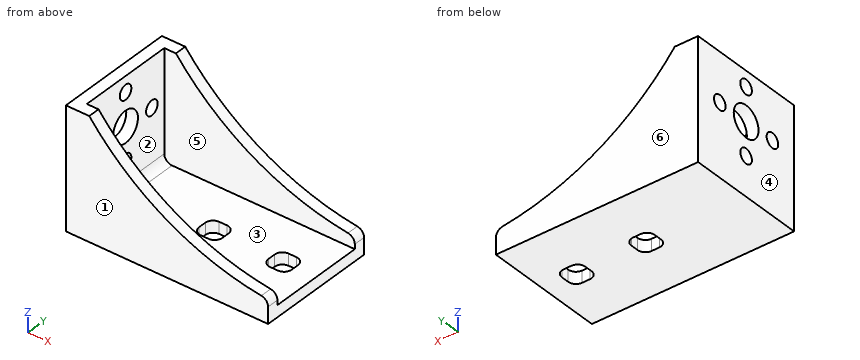
Autodesk Inventor part; units mm, degrees
ref_plane "YZ Plane" through (0, 0, 0) normal (1, 0, 0) x (0, 1, 0)
ref_plane "XZ Plane" through (0, 0, 0) normal (0, 1, 0) x (-1, 0, 0)
ref_plane "XY Plane" through (0, 0, 0) normal (0, 0, 1) x (1, 0, 0)
sketch "Sketch1" plane through (0, 0, 0) normal (0, 0, 1) x (1, 0, 0)
  line L0 (0, 0) -> (52, 0)
  line L1 (52, 0) -> (52, 31)
  line L2 (52, 31) -> (0, 31)
  line L3 (0, 31) -> (0, 0)
  line L4 (24.7, 18.5) -> (26.7, 18.5)
  line L5 (28.7, 16.5) -> (28.7, 14.5)
  line L6 (26.7, 12.5) -> (24.7, 12.5)
  line L7 (22.7, 14.5) -> (22.7, 16.5)
  arc A0 (22.7, 14.5) -> (24.7, 12.5) centre (24.7, 14.5) ccw
  arc A1 (24.7, 18.5) -> (22.7, 16.5) centre (24.7, 16.5) ccw
  arc A2 (28.7, 16.5) -> (26.7, 18.5) centre (26.7, 16.5) ccw
  arc A3 (26.7, 12.5) -> (28.7, 14.5) centre (26.7, 14.5) ccw
  line L8 (42.542, 18.5) -> (44.542, 18.5)
  line L9 (46.542, 16.5) -> (46.542, 14.5)
  line L10 (44.542, 12.5) -> (42.542, 12.5)
  line L11 (40.542, 14.5) -> (40.542, 16.5)
  arc A4 (40.542, 14.5) -> (42.542, 12.5) centre (42.542, 14.5) ccw
  arc A5 (42.542, 18.5) -> (40.542, 16.5) centre (42.542, 16.5) ccw
  arc A6 (46.542, 16.5) -> (44.542, 18.5) centre (44.542, 16.5) ccw
  arc A7 (44.542, 12.5) -> (46.542, 14.5) centre (44.542, 14.5) ccw
  point P0 (28.7, 12.5)
  point P1 (28.7, 18.5)
  point P2 (22.7, 12.5)
  point P3 (22.7, 15.5)
  point P4 (0, 15.5)
  point P5 (46.542, 12.5)
  point P6 (46.542, 18.5)
  point P7 (40.542, 12.5)
  point P8 (40.542, 15.5)
  point P9 (28.7, 15.5)
  dimension "d0" = 52
  dimension "d1" = 31
  dimension "d2" = 6
  dimension "d3" = 6
  dimension "d4" = 2
  dimension "d5" = 22.7
  dimension "d6" = 6
  dimension "d7" = 6
  dimension "d8" = 2
  dimension "d9" = 5.458
extrude "Extrusion1" add sketch "Sketch1" along normal blind 3
sketch "Sketch2" plane through (0, 0, 3) normal (0, 0, 1) x (1, 0, 0)
  line L0 (0, 31) -> (0, 0) construction
  line L1 (52, 31) -> (0, 31) construction
  line L2 (0, 0) -> (3, 0)
  line L3 (3, 0) -> (3, 31)
  line L4 (3, 31) -> (0, 31)
  line L5 (0, 31) -> (0, 0)
  dimension "d12" = 3
extrude "Extrusion2" add sketch "Sketch2" along normal blind 28
fillet "Fillet1" radius 2 1 edges at (3, 15.5, 3)
sketch "Sketch4" plane through (0, 0, 0) normal (-1, 0, 0) x (0, 0, 1)
  point P0 (0, 0)
  point P1 (18.5, 15.5)
  point P2 (31, 15.5)
  dimension "d40" = 12.5
hole "Hole1" at (0, 15.5, 18.5) direction (1, 0, 0) diameter 8 end through all
sketch "Sketch5" plane through (0, 0, 0) normal (-1, 0, 0) x (0, 0, 1)
  line L0 (0, 31) -> (0, 0) construction
  circle A0 centre (18.5, 15.5) radius 4 construction
  point P0 (18.5, 7)
  dimension "d28" = 8.5
hole "Hole2" at (0, 7, 18.5) direction (1, 0, 0) diameter 3.74 end through all
pattern_circular "Circular Pattern1" count 4 over 360 about axis through (68.0147, 15.5, 18.5) along (-1, 0, 0) of "Hole2"
sketch "Sketch7" plane through (3, 0, 31) normal (1, 0, 0) x (0, 0, -1)
  line L0 (0, 0) -> (31, 0)
  line L1 (31, 0) -> (31, 3)
  line L2 (31, 3) -> (0, 3)
  line L3 (0, 3) -> (0, 0)
  line L4 (0, 28) -> (31, 28)
  line L5 (31, 28) -> (31, 31)
  line L6 (31, 31) -> (0, 31)
  line L7 (0, 31) -> (0, 28)
  point P0 (31, 0)
  dimension "d41" = 3
  dimension "d42" = 3
extrude "Extrusion4" add sketch "Sketch7" along normal up to surface (49 mm away)
sketch "Sketch8" plane through (0, 0, 0) normal (0, -1, 0) x (1, 0, 0)
  line L0 (3, 31) -> (6, 31) construction
  line L1 (52, 3) -> (52, 6) construction
  arc A0 (6, 31) -> (52, 6) centre (58.6945, 73.1378) ccw
  line L2 (6, 31) -> (52, 31)
  line L3 (52, 31) -> (52, 6)
  point P0 (0, 0)
  dimension "d45" = 3
  dimension "d46" = 3
  dimension "d47" = 67.4708
extrude "Extrusion5" cut sketch "Sketch8" against normal up to surface (31 mm away)
fillet "Fillet2" radius 2 2 edges at (52, 1.5, 6) (52, 29.5, 6)
properties part number "sujetador del motor"
Check sheet for the modelled part. Datum: model origin and axes. Units: mm. Face numbers are marked on the shaded views. A direction names the side the tool comes from. Give positions to 0.01 mm unless a question says otherwise; leave off trailing zeros. Write each loop counter-clockwise with the first axis right and the second up, starting at its lowest first coordinate (ties: lowest second). Pieces come first, ordered by that corner, then holes. Notation, with made-up numbers: (-31.5, 37) -> (2.5, 37) arc R16 cw to (2.5, 53) -> close; hole circle Ø8 at (-16, -18.5). An arc over 180 degrees is marked (long way). Write item = value, one per line.
Item 1: Gauge pin test, flat ends, axial feed: pin 1 (5 mm diameter, centred on y = 7, z = 18.5, fed in from -X); pin 2 (1 mm diameter, centred on x = 42.5, y = 5.5, fed in from +Z); pin 3 (7.5 mm diameter, centred on y = 16.5, z = 16, fed in from +X); pin 4 (3 mm diameter, centred on y = 15.5, z = 27, fed in from -X). Record the tip position at first contact, or that the pin passes through.
Output:
pin_1 = 0
pin_2 = 3
pin_3 = 3
pin_4 = through
Item 2: Tool access check on the marked faces 1 and 2. Record the directions out of +Z, -Z, +X, -X, +Y, -Y that give a thin tool (end or side, any length) a straight path to the whole face; none if there is none.
Output:
face_1 = +Z, -Z, +X, -X, -Y
face_2 = +Z, +X
Item 3: Sectioned sample at B-B on y = 15.5. Record the boundary of the cut face in (x, z), and give its area (3 significant figures).
Output:
outline = (0, 0) -> (22.7, 0) -> (22.7, 3) -> (5, 3) arc R2 cw to (3, 5) -> (3, 8.13) -> (0, 8.13) -> close; (0, 11.87) -> (3, 11.87) -> (3, 14.5) -> (0, 14.5) -> close; (0, 22.5) -> (3, 22.5) -> (3, 25.13) -> (0, 25.13) -> close; (0, 28.87) -> (3, 28.87) -> (3, 31) -> (0, 31) -> close; (28.7, 0) -> (40.54, 0) -> (40.54, 3) -> (28.7, 3) -> close; (46.54, 0) -> (52, 0) -> (52, 3) -> (46.54, 3) -> close
area = 158 mm^2
Item 4: Sectioned sample at A-A on y = 7. Record the boundary of the cut face in (x, z), and give its area (3 significant figures).
Output:
outline = (0, 0) -> (52, 0) -> (52, 3) -> (5, 3) arc R2 cw to (3, 5) -> (3, 16.63) -> (0, 16.63) -> close; (0, 20.37) -> (3, 20.37) -> (3, 31) -> (0, 31) -> close
area = 230 mm^2
Item 5: Scan lines: probe 1 along Y at (x, z) = (1.9, 18.5); probe 2 along Z at (x, y) = (1.8, 15.5); probe 3 along Y at (x, z) = (2, 10). Record each from-to range of solid material in increasing order. Write a range as from..to.
Output:
probe_1 = 0..5.13, 8.87..11.5, 19.5..22.13, 25.87..31
probe_2 = 0..8.13, 11.87..14.5, 22.5..25.13, 28.87..31
probe_3 = 0..13.63, 17.37..31
Item 6: Sectioned sample at C-C on x = 26. Record the boundary of the cut face in (y, z), and give its area (3 significant figures).
Output:
outline = (0, 0) -> (12.5, 0) -> (12.5, 3) -> (3, 3) -> (3, 14.12) -> (0, 14.12) -> close; (18.5, 0) -> (31, 0) -> (31, 14.12) -> (28, 14.12) -> (28, 3) -> (18.5, 3) -> close
area = 142 mm^2
Item 7: Release check for a two-part mould opening along Y. For the marked faces 3, 4, 5 and 6 record: +Y half, -Y half, draft (parallel to the pull), parting line (faces both ways), or undercut.
Output:
face_3 = undercut
face_4 = draft
face_5 = undercut
face_6 = +Y half
Item 8: Sectioned sample at D-D on z = 10. Record the boundary of the cut face in (x, y), and give its area (3 significant figures).
Output:
outline = (0, 0) -> (34.91, 0) -> (34.91, 3) -> (3, 3) -> (3, 13.63) -> (0, 13.63) -> close; (0, 17.37) -> (3, 17.37) -> (3, 28) -> (34.91, 28) -> (34.91, 31) -> (0, 31) -> close
area = 273 mm^2
